Geometry: final body of the model. Coordinates: model frame, mm. A direction names the side the tool comes from. Coordinates: 2 decimals unless noted, no trailing zeros. Order: outer loops, then holes, each group sorted by start corner. A loop starts at its lowest first (then second) coordinate and runs counter-clockwise, first axis right, second up. Notation, with made-up numbers: M 60.5,83 L 95.5,83 A25 cw 95.5,110 Z; hole C -13,-4 d6. An arc over 180 degrees is marked long. One line per question, with ' | ' between items.
from build123d import *

# Parameters (mm, degrees)
SKETCH3_OUTSIDE_W  = 40.796
SKETCH3_OUTSIDE_H  = 40.796
CUT_EXTRUDE5_DEPTH = 7.62
SKETCH4_R          = 6.35
CUT_EXTRUDE6_DEPTH = 20.05


with BuildPart() as part:
    # Sketch1 → Revolve1 (revolve)
    with BuildSketch(Plane.XY):
        Polygon((0, 11.43), (-7.62, 11.43), (-7.62, 12.446), (-40.894, 12.446), (-40.894, 0), (19.05, 0), (19.05, 6.35), (0, 6.35), align=None)
    revolve(axis=Axis((-40.894, 0, 0), (1, 0, 0)))

    # Sketch3 outside → Cut-Extrude5 (cut)
    with BuildSketch(Plane(origin=(0, 0, 0), x_dir=(0, 0, -1), z_dir=(1, 0, 0))):
        Rectangle(SKETCH3_OUTSIDE_W, SKETCH3_OUTSIDE_H)
        Polygon((5.95753309, 10.31875), (-5.95753309, 10.31875), (-11.91506618, 0), (-5.95753309, -10.31875), (5.95753309, -10.31875), (11.91506618, 0), align=None, mode=Mode.SUBTRACT)
    extrude(amount=-CUT_EXTRUDE5_DEPTH, mode=Mode.SUBTRACT)

    # Sketch4 → Cut-Extrude6 (cut, through all)
    with BuildSketch(Plane(origin=(0, 0, 0), x_dir=(0, 0, -1), z_dir=(1, 0, 0))):
        Circle(SKETCH4_R)
    extrude(amount=CUT_EXTRUDE6_DEPTH, mode=Mode.SUBTRACT)


solid = part.part
1. Access query for faces 1 (the face through (-3.76, -5.1, 8.97)), 2 (the face through (-4, 10.319, 0)), 3 (the face through (-3.863, 9.905, 5.704)), 4 (the face through (-3.86, -0.01, -11.43)), 5 (the face through (-3.76, -5.22, -8.9)). Directions: +Z, -Z, +X, -X, +Y, -Y. A direction counts if a zero-diameter tool reaches every point of the face in a straight line with its end or side. Return the directions, or none.
Response values:
face 1: +Z, +X, -Y | face 2: +Z, -Z, +X, +Y | face 3: +Z, +X, +Y | face 4: -Z, +X | face 5: -Z, +X, -Y
2. Material intervals for line 1 (Y direction, x = -18, z = 0.5); line 2 (Z direction, x = -36, y = -5); line 3 (X direction, y = 6.25, z = -9.5), sorted ascending. Write a range as [from, to].
Response values:
line 1: y = [-12.44, 12.44] | line 2: z = [-11.4, 11.4] | line 3: x = [-40.89, -7.62]
3. Section A-A, the plane x = -6. Output: boundary loops of the cut face in (y, z).
Response values:
outline: M -10.32,-4.92 A11.43 ccw -9.42,-6.48 L -0.9,-11.39 A11.43 ccw 0.9,-11.39 L 9.42,-6.48 A11.43 ccw 10.32,-4.92 L 10.32,4.92 A11.43 ccw 9.42,6.48 L 0.9,11.39 A11.43 ccw -0.9,11.39 L -9.42,6.48 A11.43 ccw -10.32,4.92 Z
4. Section D-D, the plane x = -20. Output: boundary loops of the cut face in (y, z).
Response values:
outline: C 0,0 d24.89
5. Pin query (flat end, axial travel): P1, Ø3, axis at x = -22.5, z = 0.5, coming from the -Y side; P2, Ø2.5, axis at x = -3.5, z = -0.5, coming from the +Y side; P3, Ø1, axis at x = -25, z = 3, coming from the +Y side; P4, Ø5, axis at x = -19, y = 3, coming from the +Z side. Return the tip coordinate at first contact, or that it passes through.
Response values:
P1: stops at y = -12.45 | P2: stops at y = 10.32 | P3: stops at y = 12.19 | P4: stops at z = 12.44
6. Section B-B, the plane z = 0. Output: boundary loops of the cut face in (x, y), and give its area (3 significant figures).
Response values:
outline: M -40.89,-12.45 L -7.62,-12.45 L -7.62,-10.32 L 0,-10.32 L 0,10.32 L -7.62,10.32 L -7.62,12.45 L -40.89,12.45 Z | area: 986 mm^2
7. Section C-C, the plane y = 3.25. Output: boundary loops of the cut face in (x, z).
Response values:
outline: M -40.89,-12.01 L -7.62,-12.01 L -7.62,-10.04 L 0,-10.04 L 0,10.04 L -7.62,10.04 L -7.62,12.01 L -40.89,12.01 Z
